from build123d import *

# Parameters (mm, degrees)
F0_R     = 3.175
F0_R_2   = 1.5875
F1_DEPTH = 25.4


with BuildPart() as f1:
    # F0 (on Front) → F1 (new body)
    with BuildSketch(Plane.XZ):
        with BuildLine():
            ThreePointArc((44.45, -7.9375), (50.06266, -5.61266), (52.3875, 0))
            ThreePointArc((52.3875, 0), (50.06266, 5.61266), (44.45, 7.9375))
            ThreePointArc((44.45, 7.9375), (36.5125, 0), (44.45, -7.9375))
        make_face()
        with Locations((44.45, 0)):
            Circle(F0_R, mode=Mode.SUBTRACT)
        with BuildLine():
            ThreePointArc((44.45, -7.9375), (36.5125, 0), (44.45, 7.9375))
            Line((44.45, 7.9375), (17.967175, 7.9375))
            ThreePointArc((17.967175, 7.9375), (12.002232, 10.631738), (10.080201, 16.888355))
            Line((10.080201, 16.888355), (15.676557, 60.997766))
            ThreePointArc((15.676557, 60.997766), (0, 47.625), (-15.676557, 60.997766))
            Line((-15.676557, 60.997766), (-7.9375, 0))
            ThreePointArc((-7.9375, 0), (0, 7.9375), (7.9375, 0))
            ThreePointArc((7.9375, 0), (5.61266, -5.61266), (0, -7.9375))
            Line((0, -7.9375), (44.45, -7.9375))
        make_face()
        with BuildLine():
            ThreePointArc((-7.9375, 0), (-5.61266, -5.61266), (0, -7.9375))
            ThreePointArc((0, -7.9375), (5.61266, -5.61266), (7.9375, 0))
            ThreePointArc((7.9375, 0), (0, 7.9375), (-7.9375, 0))
        make_face()
        Circle(F0_R, mode=Mode.SUBTRACT)
        with BuildLine():
            Line((15.804738, 62.008062), (15.676557, 60.997766))
            ThreePointArc((15.676557, 60.997766), (15.748751, 61.501886), (15.804738, 62.008062))
        make_face()
        with BuildLine():
            ThreePointArc((-15.676557, 60.997766), (0, 47.625), (15.676557, 60.997766))
            Line((15.676557, 60.997766), (15.804738, 62.008062))
            ThreePointArc((15.804738, 62.008062), (15.857425, 62.753204), (15.875, 63.5))
            ThreePointArc((15.875, 63.5), (15.843082, 64.506168), (15.747457, 65.508289))
            ThreePointArc((15.747457, 65.508289), (0, 79.375), (-15.747457, 65.508289))
            ThreePointArc((-15.747457, 65.508289), (-15.872875, 63.75976), (-15.804738, 62.008062))
            Line((-15.804738, 62.008062), (-15.676557, 60.997766))
        make_face()
        with Locations((0, 63.5)):
            Circle(F0_R, mode=Mode.SUBTRACT)
        with BuildLine():
            ThreePointArc((-15.804738, 62.008062), (-15.748751, 61.501886), (-15.676557, 60.997766))
            Line((-15.676557, 60.997766), (-15.804738, 62.008062))
        make_face()
        with BuildLine():
            Line((-9.525, 114.3), (-15.747457, 65.508289))
            ThreePointArc((-15.747457, 65.508289), (0, 79.375), (15.747457, 65.508289))
            Line((15.747457, 65.508289), (9.525, 114.3))
            ThreePointArc((9.525, 114.3), (0, 104.775), (-9.525, 114.3))
        make_face()
        with Locations((-1.999434, 100.0252)):
            Circle(F0_R_2, mode=Mode.SUBTRACT)
        with BuildLine():
            ThreePointArc((9.525, 114.3), (0, 123.825), (-9.525, 114.3))
            ThreePointArc((-9.525, 114.3), (0, 104.775), (9.525, 114.3))
        make_face()
        with Locations((0, 114.3)):
            Circle(F0_R, mode=Mode.SUBTRACT)
    extrude(amount=F1_DEPTH)


solid = f1.part
Geometry check sheet. Reference: the model listing, model coordinates, mm. A direction names the side the tool comes from. Round coordinates to 2 decimals unless told otherwise and drop trailing zeros. Write each loop counter-clockwise with the first axis right and the second up, starting at its lowest first coordinate (ties: lowest second). Pieces come first, ordered by that corner, then holes. Notation, with made-up numbers: (86, 42) -> (127, 42) arc R17 cw to (127, 60) -> close; hole circle Ø8 at (-24, -16). An arc over 180 degrees is marked (long way). One line per item, written item: value. Start each with the question number.
(1) Scan lines: line 1 (Z direction, x = 26, y = -14.5); line 2 (Z direction, x = 45.5, y = -13.75); line 3 (X direction, y = -21, z = 39). Record each from-to range of solid material in increasing order. Write a range as [from, to].
(2) Go/stop test with flat-tipped pins: pin 1 Ø12 at (x, y) = (25.5, -3) entering from +Z; pin 2 Ø6 at (y, z) = (-4.5, 89) entering from +X; pin 3 Ø7.5 at (x, z) = (44.45, 0) entering from -Y; pin 4 Ø8 at (y, z) = (-21.5, 48) entering from -X (3 decimals). Record where each tip stops, or that it passes through.
(3) Cross-section at A-A, the plane y = -5.75. Give the number of separate pieces and of enclosed holes in the cut face, and give its area (3 significant figures).
(4) Cross-section at C-C, the plane z = 69. Record the cut outline in (x, y).
(5) Access from +Z, -Z, +X, -X, +Y, -Y to the whole of each face (thin tool, end or side, straight path). Record for faces 1 (the flat face through (31, -13, 7.938)), 2 (the cylindrical face through (12.065, -12.522, 10.561)), 3 (the cylindrical face through (-15.872, -12.522, 63.784)).
(6) Draft check along Z on faces 4 (the cylindrical face through (-0.69, -12.52, -3.1)), 5 (the flat face through (3, -25.4, 59)), 6 (the flat face through (12.68, -12.52, 89.56)), 7 (the flat face through (12.84, -12.52, 38.63)). Enter one of: +Z half, -Z half, draft (parallel to the pull), parting line (faces both ways), or undercut.
(7) Cross-section at B-B, the plane x = 29.5. Record the cut outline in (y, z).
Answer:
1. line 1: [-7.94, 7.94]
1. line 2: [-7.87, -3], [3, 7.87]
1. line 3: [-12.89, 12.89]
2. pin 1: z = 7.94
2. pin 2: x = 13.13
2. pin 3: y = -25.4
2. pin 4: x = -14.535
3. separate pieces: 1
3. enclosed holes: 5
3. area: 3,630 mm²
4. outline: (-15.3, -25.4) -> (15.3, -25.4) -> (15.3, 0) -> (-15.3, 0) -> close
5. face 1: +Z, +X, +Y, -Y
5. face 2: +X, +Y, -Y
5. face 3: -X, +Y, -Y
6. face 4: undercut
6. face 5: draft
6. face 6: +Z half
6. face 7: undercut
7. outline: (-25.4, -7.94) -> (0, -7.94) -> (0, 7.94) -> (-25.4, 7.94) -> close
